Geometry: final body of the model. Coordinates: model frame, mm. A direction names the side the tool comes from. Round coordinates to 2 decimals unless told otherwise and drop trailing zeros. Order: outer loops, then holes, each group sorted by start corner. A loop starts at its lowest first (then second) coordinate and runs counter-clockwise, first axis right, second up. Notation, with made-up numbers: M 12.5,5.5 L 65.5,5.5 A22 ccw 65.5,31.5 Z; hole C 56,88.25 d2. An arc over 180 degrees is marked long. Return JSON: item names as keys, results as strings. Group by question number.
Q1. Cut plane C-C on z = -1. Output: boundary loops of the cut face in (x, y).
Q2. Contact query for flat-ended pins moving along their axis: pin 1 (16 mm diameter, centred on x = 23, z = -17, fed in from +Y); pin 2 (22 mm diameter, centred on x = 11, y = 38.5, fed in from +Z); pin 3 (16 mm diameter, centred on x = -17.5, z = -6, fed in from +Y); pin 4 (1.5 mm diameter, centred on x = -5, y = 31.5, fed in from +Z). Output: stop coordinate, or through.
Q3. Cut plane A-A on y = 43. Output: boundary loops of the cut face in (x, z), and give its area (3 significant figures).
Q4. Access query for faces 1 (the face through (20, 40, -12)), 2 (the face through (0, 30, 0)), 3 (the face through (0, 25, -40)), 4 (the face through (-30, 25, 1)), 5 (the face through (-20, 45, 0)). Directions: +Z, -Z, +X, -X, +Y, -Y. A direction counts if a zero-diameter tool reaches every point of the face in a straight line with its end or side. Return the directions, or none.
Q5. Cut plane B-B on x = 22.5. Output: boundary loops of the cut face in (y, z), and give its area (4 significant figures).
Q6. Ray query, probe 1 along X at (y, z) = (31.5, -20.5); probe 2 along X at (y, z) = (41, 18.5); probe 3 along Y at (x, z) = (-27, -10). Return the intervals inside material, ascending.
Q7. Cut plane D-D on y = 33.5. Output: boundary loops of the cut face in (x, z), and give its area (3 significant figures).
```python
from build123d import *

# Parameters (mm, degrees)
SKETCH1_W           = 60
SKETCH1_H           = 80
BOSS_EXTRUDE1_DEPTH = 50
CUT_EXTRUDE1_DEPTH  = 70
SKETCH7_W           = 20
SKETCH7_H           = 10
CUT_EXTRUDE6_DEPTH  = 70
CUT_EXTRUDE7_DEPTH  = 70
CUT_EXTRUDE8_DEPTH  = 70


with BuildPart() as part:
    # Sketch1 → Boss-Extrude1 (new body)
    with BuildSketch(Plane(origin=(0, 0, 0), x_dir=(1, 0, 0), z_dir=(0, 1, 0))):
        Rectangle(SKETCH1_W, SKETCH1_H)
    extrude(amount=BOSS_EXTRUDE1_DEPTH)

    # Sketch2 → Cut-Extrude1 (cut)
    with BuildSketch(Plane.XY.offset(40)):
        Polygon((30, 40), (10, 40), (10, 30), (-10, 30), (-10, 50), (30, 50), align=None)
    extrude(amount=-CUT_EXTRUDE1_DEPTH, mode=Mode.SUBTRACT)

    # Sketch7 → Cut-Extrude6 (cut)
    with BuildSketch(Plane.ZY.offset(30)):
        with Locations((-10, 45)):
            Rectangle(SKETCH7_W, SKETCH7_H)
    extrude(amount=-CUT_EXTRUDE6_DEPTH, mode=Mode.SUBTRACT)

    # Sketch8 → Cut-Extrude7 (cut)
    with BuildSketch(Plane.XZ):
        Polygon((30, 40), (30, 20), (-10, 40), align=None)
    extrude(amount=-CUT_EXTRUDE7_DEPTH, mode=Mode.SUBTRACT)

    # 3DSketch6 → Cut-Extrude8 (cut, along a direction that is not the sketch's normal)
    with BuildSketch(Plane(origin=(-30, 50, 30), x_dir=(0.8241633836921342, -0.5494422557947563, -0.13736056394868917), z_dir=(0.408248290463863, 0.40824829046386274, 0.8164965809277263))):
        Polygon((0, 0), (17.856873313, 13.458531698), (27.47211279, -6.729265849), (45.328986103, 6.729265849), (40.521366365, 16.823164623), (58.378239678, 30.281696321), (72.801098893, 0), (37.087352266, -26.917063396), (9.615239476, -20.187797547), align=None)
    extrude(amount=CUT_EXTRUDE8_DEPTH, dir=(0, 0, 1), mode=Mode.SUBTRACT)


solid = part.part
```
Result sheet:
{
 "1": {"outline": "M -30,0 L 30,0 L 30,40 L 10,40 L 10,30 L -10,30 L -10,40 L -30,40 Z"},
 "2": {"pin 1": "stops at y = 40", "pin 2": "stops at z = 22.99", "pin 3": "stops at y = 50", "pin 4": "stops at z = -30"},
 "3": {"outline": "M -30,-40 L 30,-40 L 30,-30 L -10,-30 L -10,-20 L -30,-20 Z; M -30,0 L -10,0 L -10,23.5 L -30,33.5 Z", "area": "1,370 mm²"},
 "4": {"face 1": "+Z, +X, +Y", "face 2": "+Z, +Y", "face 3": "-Z, +X, -X, +Y, -Y", "face 4": "+Z, -Z, -X, +Y, -Y", "face 5": "+X, -X, +Y"},
 "5": {"outline": "M 0,-40 L 50,-40 L 50,-30 L 40,-30 L 40,8.75 L 10,23.75 L 0,23.75 Z", "area": "2,425 mm²"},
 "6": {"probe 1": "x = -30 to -10, 10 to 30", "probe 2": "x = -30 to -10", "probe 3": "y = 0 to 40"},
 "7": {"outline": "M -30,-40 L 30,-40 L 30,8.25 L 10,18.25 L 10,-30 L -10,-30 L -10,28.25 L -30,38.25 Z", "area": "2,730 mm²"}
}
